For this review, take the finished solid that the model builds, in its own axes (mm). Face numbers are marked on the shaded views. A direction names the side the tool comes from. Coordinates: 2 decimals unless noted, no trailing zeros. Write each loop counter-clockwise with the first axis right and the second up, starting at its lowest first coordinate (ties: lowest second). Pieces come first, ordered by that corner, then holes. Notation, with made-up numbers: M -18.5,8.25 L 23.5,8.25 A35 cw 23.5,40.25 Z; hole C 15.5,88 d9. An arc over 180 degrees is marked long. Return JSON: item names as keys, results as strings.
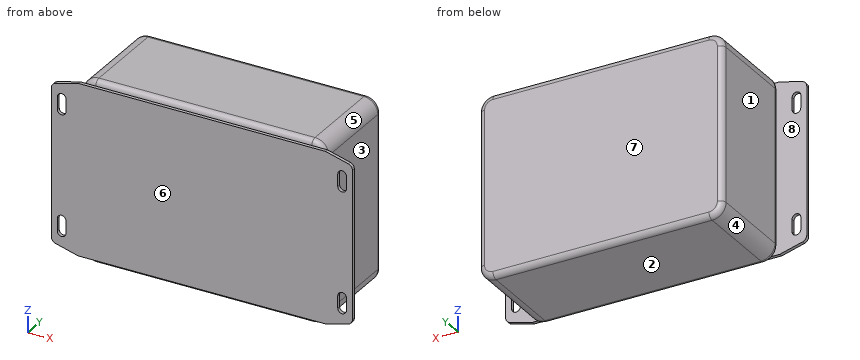
```python
from build123d import *

# Parameters (mm, degrees)
BOSS_EXTRUDE1_DEPTH = 1.524
BOSS_EXTRUDE2_DEPTH = 43.942
FILLET1_R           = 2.54


with BuildPart() as part:
    # Sketch1 → Boss-Extrude1 (new body)
    with BuildSketch(Plane(origin=(0, 0, 0), x_dir=(1, 0, 0), z_dir=(0, 1, 0))):
        with BuildLine():
            Line((-68.58, 33.629138123), (-68.58, -33.629138123))
            ThreePointArc((-68.58, -33.629138123), (-68.055117484, -35.175392152), (-66.697400375, -36.082589721))
            Line((-66.697400375, -36.082589721), (-56.3245, -38.862))
            Line((-56.3245, -38.862), (0, -38.862))
            Line((0, -38.862), (56.3245, -38.862))
            Line((56.3245, -38.862), (66.697400375, -36.082589721))
            ThreePointArc((66.697400375, -36.082589721), (68.055117484, -35.175392152), (68.58, -33.629138123))
            Line((68.58, -33.629138123), (68.58, 33.629138123))
            ThreePointArc((68.58, 33.629138123), (68.055117484, 35.175392152), (66.697400375, 36.082589721))
            Line((66.697400375, 36.082589721), (56.3245, 38.862))
            Line((56.3245, 38.862), (0, 38.862))
            Line((0, 38.862), (-56.3245, 38.862))
            Line((-56.3245, 38.862), (-66.697400375, 36.082589721))
            ThreePointArc((-66.697400375, 36.082589721), (-68.055117484, 35.175392152), (-68.58, 33.629138123))
        make_face()
        with BuildLine():
            Line((-65.8622, 24.6253), (-65.8622, 30.2387))
            ThreePointArc((-65.8622, 30.2387), (-63.881, 32.2199), (-61.8998, 30.2387))
            Line((-61.8998, 30.2387), (-61.8998, 24.6253))
            ThreePointArc((-61.8998, 24.6253), (-63.881, 22.6441), (-65.8622, 24.6253))
        make_face(mode=Mode.SUBTRACT)
        with BuildLine():
            Line((61.8998, 24.6253), (61.8998, 30.2387))
            ThreePointArc((61.8998, 30.2387), (63.881, 32.2199), (65.8622, 30.2387))
            Line((65.8622, 30.2387), (65.8622, 24.6253))
            ThreePointArc((65.8622, 24.6253), (63.881, 22.6441), (61.8998, 24.6253))
        make_face(mode=Mode.SUBTRACT)
        with BuildLine():
            Line((61.8998, -30.2387), (61.8998, -24.6253))
            ThreePointArc((61.8998, -24.6253), (63.881, -22.6441), (65.8622, -24.6253))
            Line((65.8622, -24.6253), (65.8622, -30.2387))
            ThreePointArc((65.8622, -30.2387), (63.881, -32.2199), (61.8998, -30.2387))
        make_face(mode=Mode.SUBTRACT)
        with BuildLine():
            Line((-65.8622, -30.2387), (-65.8622, -24.6253))
            ThreePointArc((-65.8622, -24.6253), (-63.881, -22.6441), (-61.8998, -24.6253))
            Line((-61.8998, -24.6253), (-61.8998, -30.2387))
            ThreePointArc((-61.8998, -30.2387), (-63.881, -32.2199), (-65.8622, -30.2387))
        make_face(mode=Mode.SUBTRACT)
    extrude(amount=BOSS_EXTRUDE1_DEPTH)


with BuildPart() as body_2:
    # Sketch2 → Boss-Extrude2 (new body)
    with BuildSketch(Plane(origin=(0, 1.524, 0), x_dir=(1, 0, 0), z_dir=(0, 1, 0))):
        with BuildLine():
            Line((55.5625, -34.925), (55.5625, 34.925))
            ThreePointArc((55.5625, 34.925), (53.702628061, 39.415128061), (49.2125, 41.275))
            Line((49.2125, 41.275), (-49.2125, 41.275))
            ThreePointArc((-49.2125, 41.275), (-53.702628061, 39.415128061), (-55.5625, 34.925))
            Line((-55.5625, 34.925), (-55.5625, -34.925))
            ThreePointArc((-55.5625, -34.925), (-53.702628061, -39.415128061), (-49.2125, -41.275))
            Line((-49.2125, -41.275), (49.2125, -41.275))
            ThreePointArc((49.2125, -41.275), (53.702628061, -39.415128061), (55.5625, -34.925))
        make_face()
    extrude(amount=BOSS_EXTRUDE2_DEPTH)

    # Fillet1
    fillet1_edges = [body_2.edges().sort_by_distance(p)[0] for p in [
        (-55.5625, 1.524, 0),
        (-53.702628061, 1.524, -39.415128061),
        (0, 1.524, -41.275),
        (53.702628061, 1.524, -39.415128061),
        (55.5625, 45.466, 0),
        (53.702628061, 45.466, 39.415128061),
        (0, 45.466, 41.275),
        (-53.702628061, 45.466, 39.415128061),
        (-55.5625, 45.466, 0),
        (-53.702628061, 45.466, -39.415128061),
        (0, 45.466, -41.275),
        (53.702628061, 45.466, -39.415128061),
        (55.5625, 1.524, 0),
        (53.702628061, 1.524, 39.415128061),
        (0, 1.524, 41.275),
        (-53.702628061, 1.524, 39.415128061),
    ]]
    fillet(fillet1_edges, radius=FILLET1_R)

    # Combine1: union part
    add(part.part)


solid = body_2.part
```
1. We need section C-C (x = 59). State the section outline as (y, z) points.
Checks:
{"outline": "M 0,-38.15 L 1.52,-38.15 L 1.52,38.15 L 0,38.15 Z"}
2. Draft analysis for pull direction Y (two halves, no side actions). For the marked faces 5, 6, 7 and 8, state which applies: +Y half, -Y half, draft (parallel to the pull), parting line (faces both ways), or undercut.
Checks:
{"face 5": "draft", "face 6": "-Y half", "face 7": "+Y half", "face 8": "undercut"}
3. Wall thickness on L1, parallel to Y at x = 59, z = 2.5; L2, parallel to X at y = 27, z = -6.5; L3, parallel to Y at x = 54, z = 27.5: over which ranges is each line inside the solid? List them lowest first. Write a range as from..to.
Checks:
{"L1": "0..1.52", "L2": "-55.56..55.56", "L3": "0..1.52, 1.72..45.27"}
4. For the marked faces 1, 2, 3 and 4, list the 3-axis set-ups (+Z, -Z, +X, -X, +Y, -Y) from which the entire face can be reached by the end or side of a thin tool; tool diameter is ignored.
Checks:
{"face 1": "+Z, -Z, -X, +Y", "face 2": "-Z, +X, -X, +Y, -Y", "face 3": "+Z, -Z, +X, +Y", "face 4": "-Z, -X, +Y"}
5. Clearance check with flat-ended pins moving along their axes: pin 1 Ø1.2 at (x, y) = (-23, 0.5) entering from -Z; pin 2 Ø2 at (y, z) = (23, 2.5) entering from +X; pin 3 Ø2 at (x, y) = (-53, 27.5) entering from +Z. State where each tip first meets the part, or that it passes through.
Checks:
{"pin 1": "z = -38.86", "pin 2": "x = 55.56", "pin 3": "z = 40.63"}
6. We need section A-A (z = 19.5). State the section outline as (x, y) points.
Checks:
{"outline": "M -68.58,0 L 68.58,0 L 68.58,1.52 L 53.02,1.52 A2.54 ccw 55.56,4.06 L 55.56,42.93 A2.54 ccw 53.02,45.47 L -53.02,45.47 A2.54 ccw -55.56,42.93 L -55.56,4.06 A2.54 ccw -53.02,1.52 L -68.58,1.52 Z"}
